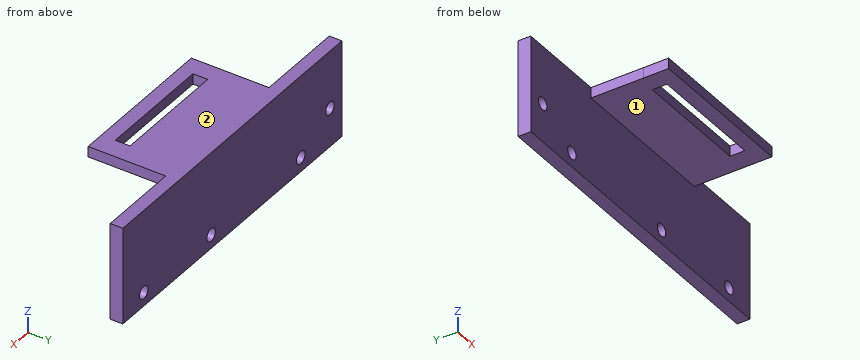
```python
from build123d import *

# Parameters (mm, degrees)
SKETCH_1_W                = 78
SKETCH_1_H                = 15
EXTRUDE_1_DEPTH           = 3
SKETCH_3_R                = 1.5
CUT_EXTRUDE_1_DEPTH       = 3
SKETCH_4_R                = 6
EXTRUDE_2_DEPTH           = 18
SKETCH_5_R                = 4.5
CUT_EXTRUDE_2_DEPTH       = 21
F_2_0MM_2_D               = 3
F_2_0MM_2_DEPTH           = 4.5
F_2_0MM_2_TIP             = 1.5
F_2_0MM_2_ON_FACE_2_D     = 3
F_2_0MM_2_ON_FACE_2_DEPTH = 4.5
F_2_0MM_2_ON_FACE_2_TIP   = 1.5
SKETCH_10_W               = 6
SKETCH_10_H               = 10
CUT_EXTRUDE_3_DEPTH       = 7
SKETCH_13_W               = 19.835687411
SKETCH_13_H               = 21.610205193
CUT_EXTRUDE_4_DEPTH       = 20
SKETCH_14_W               = 11.523038103
SKETCH_14_H               = 10.49031299
EXTRUDE_3_DEPTH           = 3
SKETCH_18_W               = 78
SKETCH_18_H               = 8
EXTRUDE_4_DEPTH           = 3
SKETCH_19_W               = 36.767904102
SKETCH_19_H               = 2.5
EXTRUDE_5_DEPTH           = 12.5
SKETCH_23_R               = 1.65
CUT_EXTRUDE_6_DEPTH       = 12.5
SKETCH_25_W               = 4.236607592
SKETCH_25_H               = 5.36409187
EXTRUDE_7_DEPTH           = 2.5
SKETCH_26_R               = 1.6
CUT_EXTRUDE_7_DEPTH       = 2.5
SKETCH_27_W               = 21.346012392
SKETCH_27_H               = 6.594354882
EXTRUDE_8_DEPTH           = 2.5
SKETCH_28_W               = 36.767231154
SKETCH_28_H               = 5.91819544
EXTRUDE_9_DEPTH           = 2.5
SKETCH_29_W               = 27.660340415
SKETCH_29_H               = 3.5
CUT_EXTRUDE_9_DEPTH       = 2.5


with BuildPart() as part:
    # 草图1 → 凸台-拉伸1 (new body)
    with BuildSketch(Plane(origin=(0, 0, 0), x_dir=(1, 0, 0), z_dir=(0, 1, 0))):
        Rectangle(SKETCH_1_W, SKETCH_1_H)
    extrude(amount=EXTRUDE_1_DEPTH)

    # 草图3 → 切除-拉伸1 (cut)
    with BuildSketch(Plane(origin=(0, 3, 0), x_dir=(1, 0, 0), z_dir=(0, 1, 0))):
        with Locations(Location((-34.76, -1.72, 0), (0, 0, 270))):
            Circle(SKETCH_3_R)
        with Locations(Location((-24.35, 4.1, 0), (0, 0, 270))):
            Circle(SKETCH_3_R)
        with Locations(Location((31.56, 4.221692081, 0), (0, 0, 270))):
            Circle(SKETCH_3_R)
        with Locations(Location((7.56, 4.221692081, 0), (0, 0, 270))):
            Circle(SKETCH_3_R)
    extrude(amount=-CUT_EXTRUDE_1_DEPTH, mode=Mode.SUBTRACT)

    # 草图4 → 凸台-拉伸2 (add)
    with BuildSketch(Plane(origin=(0, 3, 0), x_dir=(1, 0, 0), z_dir=(0, 1, 0))):
        with Locations(Location((-3, -1.234165229, 0), (0, 0, 270))):
            Circle(SKETCH_4_R)
    extrude(amount=EXTRUDE_2_DEPTH)

    # 草图5 → 切除-拉伸2 (cut)
    with BuildSketch(Plane(origin=(0, 21, 0), x_dir=(1, 0, 0), z_dir=(0, 1, 0))):
        with Locations(Location((-3, -1.234165229, 0), (0, 0, 270))):
            Circle(SKETCH_5_R)
    extrude(amount=-CUT_EXTRUDE_2_DEPTH, mode=Mode.SUBTRACT)

    # Ø2.0mm 暗销孔2
    with Locations(Plane(origin=(-7.901331048, 17.342107422, 4.694938836), x_dir=(-0.576795601176, 0, -0.816888507977), z_dir=(-0.816888507977, 0, 0.576795601176))):
        with Locations((0, 0)):
            Hole(F_2_0MM_2_D / 2, depth=F_2_0MM_2_DEPTH)
            with Locations((0, 0, -(F_2_0MM_2_DEPTH + F_2_0MM_2_TIP / 2))):  # 90° drill point
                Cone(0, F_2_0MM_2_D / 2, F_2_0MM_2_TIP, mode=Mode.SUBTRACT)

    # Ø2.0mm 暗销孔2 on face 2
    with Locations(Plane(origin=(1.071764877, 17.164817099, 5.641061052), x_dir=(0.734483043181, 0, -0.678627039897), z_dir=(0.678627039897, 0, 0.734483043181))):
        with Locations((0, 0)):
            Hole(F_2_0MM_2_ON_FACE_2_D / 2, depth=F_2_0MM_2_ON_FACE_2_DEPTH)
            with Locations((0, 0, -(F_2_0MM_2_ON_FACE_2_DEPTH + F_2_0MM_2_ON_FACE_2_TIP / 2))):  # 90° drill point
                Cone(0, F_2_0MM_2_ON_FACE_2_D / 2, F_2_0MM_2_ON_FACE_2_TIP, mode=Mode.SUBTRACT)

    # 草图10 → 切除-拉伸3 (cut)
    with BuildSketch(Plane(origin=(0, 0, -7.5), x_dir=(-1, 0, 0), z_dir=(0, 0, -1))):
        with Locations((3, 8)):
            Rectangle(SKETCH_10_W, SKETCH_10_H)
    extrude(amount=-CUT_EXTRUDE_3_DEPTH, mode=Mode.SUBTRACT)

    # 草图13 → 切除-拉伸4 (cut)
    with BuildSketch(Plane(origin=(0, 0, -7.5), x_dir=(-1, 0, 0), z_dir=(0, 0, -1))):
        with Locations((3.314421038, 13.805102597)):
            Rectangle(SKETCH_13_W, SKETCH_13_H)
    extrude(amount=-CUT_EXTRUDE_4_DEPTH, mode=Mode.SUBTRACT)

    # 草图14 → 凸台-拉伸3 (add)
    with BuildSketch(Plane(origin=(0, 3, 0), x_dir=(1, 0, 0), z_dir=(0, 1, 0))):
        with Locations((-2.989467433, -1.263493391)):
            Rectangle(SKETCH_14_W, SKETCH_14_H)
    extrude(amount=-EXTRUDE_3_DEPTH)

    # 草图18 → 凸台-拉伸4 (add)
    with BuildSketch(Plane.XZ):
        with Locations((0, 11.5)):
            Rectangle(SKETCH_18_W, SKETCH_18_H)
    extrude(amount=-EXTRUDE_4_DEPTH)

    # 草图19 → 凸台-拉伸5 (add)
    with BuildSketch(Plane.XZ):
        with Locations((0.839237194, 14.25)):
            Rectangle(SKETCH_19_W, SKETCH_19_H)
    extrude(amount=EXTRUDE_5_DEPTH)

    # 草图23 → 切除-拉伸6 (cut)
    with BuildSketch(Plane(origin=(0, 0, 13), x_dir=(-1, 0, 0), z_dir=(0, 0, -1))):
        with Locations((-8.603189245, -6.05592298)):
            Circle(SKETCH_23_R)
        with Locations((2.596810755, -6.05592298)):
            Circle(SKETCH_23_R)
    extrude(amount=-CUT_EXTRUDE_6_DEPTH, mode=Mode.SUBTRACT)

    # 草图25 → 凸台-拉伸7 (add)
    with BuildSketch(Plane(origin=(0, 0, 13), x_dir=(-1, 0, 0), z_dir=(0, 0, -1))):
        with Locations((2.330668631, -6.426480946)):
            Rectangle(SKETCH_25_W, SKETCH_25_H)
    extrude(amount=-EXTRUDE_7_DEPTH)

    # 草图26 → 切除-拉伸7 (cut)
    with BuildSketch(Plane(origin=(0, 0, 13), x_dir=(-1, 0, 0), z_dir=(0, 0, -1))):
        with Locations((4.196810755, -6.05592298)):
            Circle(SKETCH_26_R)
    extrude(amount=-CUT_EXTRUDE_7_DEPTH, mode=Mode.SUBTRACT)

    # 草图27 → 凸台-拉伸8 (add)
    with BuildSketch(Plane(origin=(0, 0, 13), x_dir=(-1, 0, 0), z_dir=(0, 0, -1))):
        with Locations((-2.379316694, -6.691741876)):
            Rectangle(SKETCH_27_W, SKETCH_27_H)
    extrude(amount=-EXTRUDE_8_DEPTH)

    # 草图28 → 凸台-拉伸9 (add)
    with BuildSketch(Plane(origin=(0, 0, 13), x_dir=(-1, 0, 0), z_dir=(0, 0, -1))):
        with Locations((-0.839573668, -15.45909772)):
            Rectangle(SKETCH_28_W, SKETCH_28_H)
    extrude(amount=-EXTRUDE_9_DEPTH)

    # 草图29 → 切除-拉伸9 (cut)
    with BuildSketch(Plane(origin=(0, 0, 13), x_dir=(-1, 0, 0), z_dir=(0, 0, -1))):
        with Locations((-0.633763758, -13.394190827)):
            Rectangle(SKETCH_29_W, SKETCH_29_H)
    extrude(amount=-CUT_EXTRUDE_9_DEPTH, mode=Mode.SUBTRACT)


solid = part.part
```
The listing builds one solid part. Answer for the finished solid, in the listing's coordinates (mm). Face numbers are marked on the shaded views. A direction names the side the tool comes from. Coordinates: 2 decimals unless noted, no trailing zeros. Write each loop counter-clockwise with the first axis right and the second up, starting at its lowest first coordinate (ties: lowest second). Pieces come first, ordered by that corner, then holes.
Q1. Find the intervals of material crossed by line 1 along Y through (x, z) = (13.5, 13.25); line 2 along X through (y, z) = (1.85, -4.1); line 3 along X through (y, z) = (1.5, -3), in increasing order.
Returned:
line 1: y = -18.42 to -15.14, -11.64 to 3
line 2: x = -39 to -25.85, -22.85 to 6.06, 9.06 to 30.06, 33.06 to 39
line 3: x = -39 to -25.37, -23.33 to 6.69, 8.43 to 30.69, 32.43 to 39
Q2. Given P1, Ø3, axis at y = -5.5, z = 15, coming from the -X side; P2, Ø4, axis at x = 2.5, y = -9, coming from the -Z side; P3, Ø1.8, axis at x = -24.35, z = -4.1, coming from the +Y side; P4, Ø8, axis at y = -14, z = 10, coming from the +X side, each flat-ended and moving along its own axis, determine where each tip first touches the part or whether it passes through.
Returned:
P1: stops at x = -17.54
P2: stops at z = 13
P3: passes through
P4: stops at x = 19.22
Q3. Section D-D, the plane x = 31.56 is taken. Write down the section's boundary in (y, z).
Returned:
outline: (0, -7.5) - (3, -7.5) - (3, -5.72) - (0, -5.72) - close; (0, -2.72) - (3, -2.72) - (3, 15.5) - (0, 15.5) - close
Q4. Which of the six approach directions +Z, -Z, +X, -X, +Y, -Y give full straight-line access (tool end or side, diameter ignored) to the marked faces 1 and 2?
Returned:
face 1: -Z, +X, -X, -Y
face 2: +Z, +X, -X, +Y, -Y
Q5. Section C-C, the plane z = 1.72 is taken. Write down the section's boundary in (x, y), then the cut area to 3 significant figures.
Returned:
outline: (-39, 0) - (-36.26, 0) - (-36.26, 3) - (-39, 3) - close; (-33.26, 0) - (39, 0) - (39, 3) - (-33.26, 3) - close
area: 225 mm2
Q6. Section B-B, the plane x = 7.56 is taken. Write down the section's boundary in (y, z).
Returned:
outline: (-18.42, 13) - (-15.14, 13) - (-15.14, 15.5) - (-18.42, 15.5) - close; (-11.64, 13) - (0, 13) - (0, -2.72) - (3, -2.72) - (3, 15.5) - (-11.64, 15.5) - close; (0, -7.5) - (3, -7.5) - (3, -5.72) - (0, -5.72) - close
Q7. Section A-A, the plane y = 1.25 is taken. Write down the section's boundary in (x, z).
Returned:
outline: (-39, -7.5) - (39, -7.5) - (39, 15.5) - (-39, 15.5) - close; hole circle Ø3 at (-34.76, 1.72); hole circle Ø3 at (-24.35, -4.1); hole circle Ø3 at (7.56, -4.22); hole circle Ø3 at (31.56, -4.22)
